Autodesk Inventor part; units mm, degrees
ref_plane "YZ Plane" through (0, 0, 0) normal (1, 0, 0) x (0, 1, 0)
ref_plane "XZ Plane" through (0, 0, 0) normal (0, 1, 0) x (-1, 0, 0)
ref_plane "XY Plane" through (0, 0, 0) normal (0, 0, 1) x (1, 0, 0)
sketch "Sketch1" plane through (0, 0, 0) normal (0, 0, 1) x (1, 0, 0)
  line L0 (-750, 51.765) -> (750, 51.765)
  line L1 (750, 51.765) -> (750, 0)
  line L2 (750, 0) -> (-750, 0)
  line L3 (-750, 0) -> (-750, 51.765)
  point P0 (0, 0)
  point P1 (0, 0)
  dimension "d0" = 1500
  dimension "d1" = 51.765
extrude "Plate1" add sketch "Sketch1" along normal blind 2
sketch "Sketch2" plane through (750, 2, 0) normal (0, -1, 0) x (1, 0, 0)
  line L0 (-1500, 0) -> (0, 0)
  line L1 (0, 0) -> (0, 20)
  line L2 (0, 20) -> (-1500, 20)
  line L3 (-1500, 20) -> (-1500, 0)
edge flange "Flange1" height 20 angle 90 thickness 2 bend radius 2.75 thickness toward (0, -1, 0) relief round relief width 2 relief depth 1 edges at (0, 0, 2) wall of the first edge with corners at (-750, 2, 0) (750, 2, 0) (750, 2, 20) (-750, 2, 20)
bend "Bend1"
corner "Corner1"
sketch "Sketch5" plane through (0, 0, 0) normal (0, 0, -1) x (-1, 0, 0)
  line L0 (750, 51.765) -> (-750, 51.765)
  line L1 (-1, 30) -> (-1, 51.765)
  line L2 (750, 0) -> (-750, 0)
  line L3 (-1, 30) -> (1, 30)
  line L4 (1, 30) -> (1, 51.765)
  point P0 (0, 0)
  point P1 (0, 30)
  point P2 (0, 0)
  dimension "d27" = 2
  dimension "d29" = 30
extrude "Extrusion1" cut sketch "Sketch5" against normal through all
pattern_linear "Rectangular Pattern1" count 3 spacing 500 along (1, 0, 0) of "Extrusion1" first direction both ways yes
sketch "Sketch6" plane through (0, 0, 0) normal (0, 0, -1) x (-1, 0, 0)
  line L0 (-750, 51.765) -> (-750, 4.75)
  circle A0 centre (-750, 51.765) radius 22.5
  line L1 (-750, 51.765) -> (750, 51.765)
  line L2 (-499, 30) -> (-501, 30) construction
  line L3 (-499, 30) -> (-1, 30) construction
  line L4 (-1, 30) -> (-1, 51.765) construction
  line L5 (-1, 51.765) -> (-499, 51.765)
  circle A1 centre (-250, 51.765) radius 22.5
  point P0 (0, 0)
  point P1 (-727.5, 51.765)
  point P2 (-750, 29.265)
  point P3 (-250, 30)
  point P4 (-227.5, 51.765)
  point P5 (-272.5, 51.765)
  dimension "d24" = 45
extrude "Extrusion2" cut sketch "Sketch6" against normal through all contours L1 A0 L0 | L1 A1 picked at (-748.3311, 36.953) picked at (-248.2369, 40.8343)
mirror "Mirror1" about plane through (0, 0, 0) normal (1, 0, 0) of "Extrusion2"
sketch "Sketch7" plane through (0, 0, 2) normal (0, 0, 1) x (1, 0, 0)
  arc A0 (-750, 29.265) -> (-727.5, 51.765) centre (-750, 51.765) ccw
  line L0 (-750, 4.75) -> (-750, 29.265)
  line L1 (-750, 4.75) -> (750, 4.75)
  line L2 (750, 29.265) -> (750, 4.75)
  arc A1 (727.5, 51.765) -> (750, 29.265) centre (750, 51.765) ccw
  line L3 (501, 51.765) -> (727.5, 51.765)
  line L4 (501, 51.765) -> (501, 30)
  line L5 (501, 30) -> (499, 30)
  line L6 (499, 30) -> (499, 51.765)
  line L7 (1, 51.765) -> (227.5, 51.765)
  line L8 (1, 51.765) -> (1, 30)
  line L9 (1, 30) -> (-1, 30)
  line L10 (-1, 30) -> (-1, 51.765)
  line L11 (-499, 51.765) -> (-272.5, 51.765)
  line L12 (-499, 51.765) -> (-499, 30)
  line L13 (-499, 30) -> (-501, 30)
  line L14 (-501, 30) -> (-501, 51.765)
  line L15 (-727.5, 51.765) -> (-501, 51.765)
  line L16 (649, 50.765) -> (651, 50.765)
  line L17 (651, 50.765) -> (651, 51.765)
  line L18 (651, 51.765) -> (649, 51.765)
  line L19 (649, 51.765) -> (649, 50.765)
  line L20 (650, 4.75) -> (650, 51.765) construction
  line L21 (272.5, 51.765) -> (499, 51.765)
  arc A2 (227.5, 51.765) -> (272.5, 51.765) centre (250, 51.765) ccw
  line L22 (-227.5, 51.765) -> (-1, 51.765)
  arc A3 (-272.5, 51.765) -> (-227.5, 51.765) centre (-250, 51.765) ccw
  point P0 (0, 0)
  point P1 (650, 50.765)
  point P2 (649, 51.265)
  point P3 (650, 28.2575)
  dimension "d30" = 2
  dimension "d31" = 1
  dimension "d33" = 100
extrude "Extrusion3" [suppressed]
mirror "Mirror2" [suppressed]
sketch "Sketch9" plane through (0, 0, 2) normal (0, 0, 1) x (1, 0, 0)
  line L0 (494, 46.765) -> (494, 34.765) construction
  line L1 (494, 34.765) -> (294, 34.765) construction
  line L2 (294, 34.765) -> (294, 46.765) construction
  line L3 (294, 46.765) -> (494, 46.765) construction
  line L4 (499, 30) -> (499, 51.765)
  line L5 (1, 51.765) -> (499, 51.765)
  point P0 (0, 0)
  dimension "d38" = 200
  dimension "d39" = 12
  dimension "d42" = 5
  dimension "d43" = 5
mark "Mark3"
equation "\"d1\" = Стрингер_1"
equation "\"d27\" = d18"
equation "\"d29\" = Стрингер_глубина_паза"
equation "\"d43\" = d42"
equation "\"d2\" = Thickness"
equation "\"d3\" = BendReliefWidth"
equation "\"d4\" = BendReliefDepth"
equation "\"d5\" = MinimumRemnant"
equation "\"d6\" = TransitionRadius"
equation "\"d9\" = BendRadius"
equation "\"d10\" = CornerReliefSize"
equation "\"d11\" = GapSize"
equation "\"d12\" = JacobiRadiusSize"
equation "\"BendReliefWidth\" = Thickness"
equation "\"BendReliefDepth\" = 0.5 * Thickness"
equation "\"CornerReliefSize\" = 4 * Thickness"
equation "\"MinimumRemnant\" = 2 * Thickness"
equation "\"TransitionRadius\" = BendRadius"
equation "\"JacobiRadiusSize\" = BendRadius"
equation "\"GapSize\" = Thickness"
equation "\"d18\" = Thickness"
equation "\"qqqqqq\" = 67.35706"
properties part number "MSC 061 stringer back ^" material "Stainless Steel"
The model under review builds one solid part; all positions refer to its coordinate system, in mm. A direction names the side the tool comes from. Round coordinates to 2 decimals unless told otherwise and drop trailing zeros. Loops run counter-clockwise (first coordinate to the right, second up) from the corner with the lowest first, then second, coordinate; pieces in that order, holes last. Notation, with made-up numbers: M 11,78 L 35,78 A19 cw 35,96 Z; hole C 32.5,42 d9. An arc over 180 degrees is marked long. Answer as a JSON object with one key per item and string values.
Item 1: Clearance check with flat-ended pins moving along their axes: P1, Ø1.6, axis at x = 500, z = 1, coming from the +Y side; P2, Ø2, axis at y = 44, z = 1.5, coming from the -X side; P3, Ø2, axis at y = 36, z = 1, coming from the +X side. State where each tip first meets the part, or that it passes through.
Check sheet entries:
{"P1": "y = 30", "P2": "x = -729.28", "P3": "x = 734.99"}
Item 2: We need section B-B, the plane z = 8.5. State the section outline as (x, y) points, and give its area (3 significant figures).
Check sheet entries:
{"outline": "M -750,0 L 750,0 L 750,2 L -750,2 Z", "area": "3,000 mm2"}
Item 3: We need section D-D, the plane x = -157.5. State the section outline as (y, z) points (3 decimals).
Check sheet entries:
{"outline": "M 0,4.75 A4.75 ccw 4.75,0 L 51.765,0 L 51.765,2 L 4.75,2 A2.75 cw 2,4.75 L 2,20 L 0,20 Z"}
Item 4: For line 1 along Z through (x, y) = (188.5, 38); line 2 along Y through (x, z) = (453, 2.25), list the stretches that pass through material, from the lowest coordinate up.
Check sheet entries:
{"line 1": "0 to 2", "line 2": "0.71 to 3.6"}
Item 5: We need section A-A, the plane x = 250. State the section outline as (y, z) points (3 decimals).
Check sheet entries:
{"outline": "M 0,4.75 A4.75 ccw 4.75,0 L 29.265,0 L 29.265,2 L 4.75,2 A2.75 cw 2,4.75 L 2,20 L 0,20 Z"}
Item 6: Tool access review of faces 1 (the face through (-10, 29, 2)), 2 (the face through (-10, 29, 0)): name each direction out of +Z, -Z, +X, -X, +Y, -Y from which nothing blocks a thin tool from reaching the whole face with its end or side.
Check sheet entries:
{"face 1": "+Z, +X, -X, +Y", "face 2": "-Z, +X, -X, +Y, -Y"}
